```python
from build123d import *

# Parameters (mm, degrees)
BOSS_EXTRUDE1_DEPTH = 1.6
SKETCH2_R           = 1
CUT_EXTRUDE1_DEPTH  = 2.6
CUT_EXTRUDE2_DEPTH  = 0.8


with BuildPart() as part:
    # Sketch1 → Boss-Extrude1 (new body)
    with BuildSketch(Plane(origin=(0, 0, 0), x_dir=(1, 0, 0), z_dir=(0, 1, 0))):
        with BuildLine():
            Line((-9, 26.094133447), (-3.675272118, 45.890528901))
            ThreePointArc((-3.675272118, 45.890528901), (-2.266272493, 49.203119101), (0, 52))
            Line((0, 52), (-1.5, 38.573765251))
            Line((-1.5, 38.573765251), (0, 37))
            Line((0, 37), (-6.5, 0))
            ThreePointArc((-6.5, 0), (-7.739867281, 0.785826002), (-8.065788204, 2.217108271))
            Line((-8.065788204, 2.217108271), (-4.822378182, 21.445480314))
            Line((-4.822378182, 21.445480314), (-9, 26.094133447))
        make_face()
    extrude(amount=BOSS_EXTRUDE1_DEPTH)

    # Sketch2 → Cut-Extrude1 (cut, through all)
    with BuildSketch(Plane(origin=(0, 1.6, 0), x_dir=(1, 0, 0), z_dir=(0, 1, 0))):
        with Locations((-4.6, 29.094133447)):
            Circle(SKETCH2_R)
    extrude(amount=-CUT_EXTRUDE1_DEPTH, mode=Mode.SUBTRACT)

    # Sketch4 → Cut-Extrude2 (cut)
    with BuildSketch(Plane.XZ):
        Polygon((-5.441038935, -22.133895727), (-15.455204314, -22.133895727), (-15.455204314, -68.130413952), (6.621463741, -68.130413952), (6.621463741, -27.758733102), align=None)
    extrude(amount=-CUT_EXTRUDE2_DEPTH, mode=Mode.SUBTRACT)


solid = part.part
```
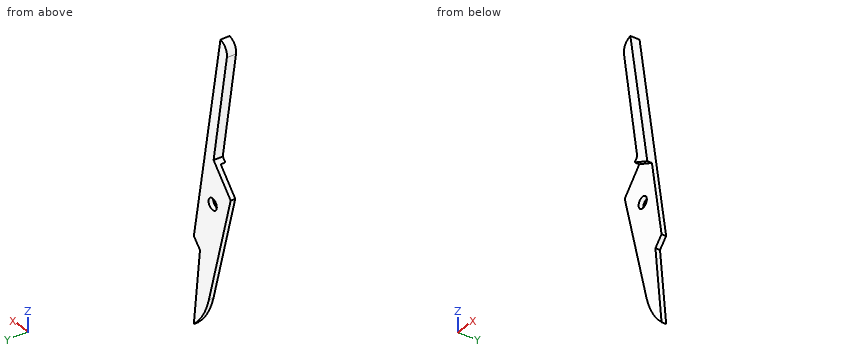
Input: part model. Units: mm. Frame: model coordinates. Coordinates: 2 decimals unless noted, no trailing zeros. Order: outer loops, then holes, each group sorted by start corner. A loop starts at its lowest first (then second) coordinate and runs counter-clockwise, first axis right, second up. Notation, with made-up numbers: (48.25, -34) - (75.25, -34) arc R26 ccw to (75.25, -7) - close; hole circle Ø9 at (14, 1.5). An arc over 180 degrees is marked (long way). Put each result on its own line as item: value.
1. Cut plane C-C on z = -6.5. Return the cut outline in (x, y).
Report:
outline: (-7.34, 0) - (-5.36, 0) - (-5.36, 1.6) - (-7.34, 1.6) - close
2. Line query: line 1 along Y through (x, z) = (-2, -43.5); line 2 along X through (y, z) = (1.1, -27); line 3 along X through (y, z) = (0.2, -13). Output: solid intervals per line, ascending.
Report:
line 1: y = 0.8 to 1.6
line 2: x = -8.76 to -1.76
line 3: x = -6.25 to -4.22
3. Contact query for a flat-ended pin moving along its axis: pin 1 Ø2.5 at (x, z) = (-4.6, -29.09) entering from -Y. Output: stop coordinate, or through.
Report:
pin 1: stops at y = 0.8
4. Cut plane D-D on z = -20. Return the cut outline in (x, y), then the cut area to 3 significant figures.
Report:
outline: (-5.07, 0) - (-2.99, 0) - (-2.99, 1.6) - (-5.07, 1.6) - close
area: 3.33 mm2
5. Cut plane B-B on y = 1.15. Return the cut outline in (x, z), then the cut area to 3 significant figures.
Report:
outline: (-9, -26.09) - (-3.68, -45.89) arc R12.95 ccw to (0, -52) - (-1.5, -38.57) - (0, -37) - (-6.5, 0) arc R1.93 ccw to (-8.07, -2.22) - (-4.82, -21.45) - close; hole circle Ø2 at (-4.6, -29.09)
area: 178 mm2
6. Cut plane A-A on x = -0.75. Return the cut outline in (y, z), then the cut area to 3 significant figures.
Report:
outline: (0.8, -51.24) - (1.6, -51.24) - (1.6, -45.29) - (0.8, -45.29) - close; (0.8, -37.79) - (1.6, -37.79) - (1.6, -32.73) - (0.8, -32.73) - close
area: 8.81 mm2
